Could you check a few things on this model? Use its own coordinates, in mm. A direction names the side the tool comes from. Coordinates: 2 decimals unless noted, no trailing zeros. Order: outer loops, then holes, each group sorted by start corner. A loop starts at its lowest first (then second) coordinate and runs counter-clockwise, first axis right, second up.
```python
from build123d import *

# Parameters (mm, degrees)
SKETCH1_W           = 200
SKETCH1_H           = 110
BOSS_EXTRUDE1_DEPTH = 3.175
CUT_EXTRUDE1_REACH  = 5.175
CUT_EXTRUDE2_REACH  = 5.175
SKETCH4_W           = 6.35
SKETCH4_H           = 25
CUT_EXTRUDE3_DEPTH  = 3.175
SKETCH5_R           = 3.175
CUT_EXTRUDE4_DEPTH  = 10
LPATTERN1_COUNT     = 3
LPATTERN1_PITCH     = 30


with BuildPart() as part:
    # Sketch1 → Boss-Extrude1 (new body)
    with BuildSketch(Plane(origin=(0, 0, 0), x_dir=(1, 0, 0), z_dir=(0, 1, 0))):
        with Locations((100, 55)):
            Rectangle(SKETCH1_W, SKETCH1_H)
    extrude(amount=BOSS_EXTRUDE1_DEPTH)

    # Sketch2 → Cut-Extrude1 (cut, up to next)
    with BuildSketch(Plane(origin=(0, 3.175, 0), x_dir=(1, 0, 0), z_dir=(0, 1, 0)), mode=Mode.PRIVATE) as cut_extrude1_sk1:
        Polygon((194, 22.467727943), (174.625274195, 3.093002139), (170.135146135, 7.583130199), (189.509871939, 26.957856004), align=None)
    cut_extrude1_tool1 = extrude(cut_extrude1_sk1.sketch, amount=-CUT_EXTRUDE1_REACH, mode=Mode.PRIVATE) & part.part
    add(cut_extrude1_tool1.solids().sort_by_distance((182.067573, 3.175, -15.025429))[0], mode=Mode.SUBTRACT)

    # Sketch3 → Cut-Extrude2 (cut, up to next)
    with BuildSketch(Plane(origin=(0, 3.175, 0), x_dir=(1, 0, 0), z_dir=(0, 1, 0)), mode=Mode.PRIVATE) as cut_extrude2_sk1:
        Polygon((168.509871939, 71.151828996), (179.151828996, 60.509871939), (183.641957057, 65), (173, 75.641957057), align=None)
    cut_extrude2_tool1 = extrude(cut_extrude2_sk1.sketch, amount=-CUT_EXTRUDE2_REACH, mode=Mode.PRIVATE) & part.part
    add(cut_extrude2_tool1.solids().sort_by_distance((176.075914, 3.175, -68.075914))[0], mode=Mode.SUBTRACT)

    # Sketch4 → Cut-Extrude3 (cut)
    with BuildSketch(Plane(origin=(0, 3.175, 0), x_dir=(1, 0, 0), z_dir=(0, 1, 0))):
        with Locations((8.175, 24.889181128)):
            Rectangle(SKETCH4_W, SKETCH4_H)
    cut_extrude3 = extrude(amount=-CUT_EXTRUDE3_DEPTH, mode=Mode.SUBTRACT)

    # Sketch5 → Cut-Extrude4 (cut)
    with BuildSketch(Plane(origin=(0, 3.175, 0), x_dir=(1, 0, 0), z_dir=(0, 1, 0))):
        with Locations((8, 102)):
            Circle(SKETCH5_R)
        with Locations((192, 102)):
            Circle(SKETCH5_R)
        with Locations((192, 8)):
            Circle(SKETCH5_R)
        with Locations((8, 8)):
            Circle(SKETCH5_R)
    extrude(amount=-CUT_EXTRUDE4_DEPTH, mode=Mode.SUBTRACT)

    # LPattern1: Cut-Extrude3 ×3
    with Locations(*[(i * LPATTERN1_PITCH, 0, 0) for i in range(1, LPATTERN1_COUNT)]):
        add(cut_extrude3, mode=Mode.SUBTRACT)


solid = part.part
```
Item 1: Which directions (+Z, -Z, +X, -X, +Y, -Y) give clear straight access to the entire face, cutting with the end or side of a thin tool? Please do faces 3 (the face through (99, 0, -56)), 4 (the face through (172.41, 1.61, -5.31)).
Item 2: Suppose I cut it at D-D (z = -35). List the corners of the cut face in (x, y) for me (3 decimals), and give its area (3 significant figures).
Item 3: I need wall thicknesses on line 1 (X direction, y = 2.4, z = -101.5); line 2 (X direction, y = 1.8, z = -102) (3 decimals); line 3 (Z direction, x = 192, y = 1.4) (3 decimals). Which ranges of each line are inside material? Lowest first, please.
Item 4: Suppose I cut it at B-B (x = 8). List the corners of the cut face in (y, z) for me (3 decimals).
Item 5: For pin 1 Ø1 at (x, y) = (7, 1) entering from +Z; pin 2 Ø5 at (x, z) = (192, -8) entering from +Y, each with a flat end and sliding along its axis, tell me the tip position at first contact or that it passes through.
Item 6: Thinking about a two-plate mould opening in Z: for faces 1 (the face through (99, 3.175, -56)), 2 (the face through (184.45, 1.61, -12.92)), which applies, +Z half, -Z half, draft (parallel to the pull), parting line (faces both ways), or undercut?
Item 7: Suppose I cut it at A-A (z = -102). List the corners of the cut face in (x, y) for me (3 decimals).
Item 8: Suppose I cut it at C-C (y = 1.35). Count the separate pieces of the cut face and the enclosed holes in it, and give its area (3 significant figures).
Geometry results:
1. face 3: +Z, -Z, +X, -X, -Y
1. face 4: +Y, -Y
2. outline: (0, 0) - (5, 0) - (5, 3.175) - (0, 3.175) - close; (11.35, 0) - (35, 0) - (35, 3.175) - (11.35, 3.175) - close; (41.35, 0) - (65, 0) - (65, 3.175) - (41.35, 3.175) - close; (71.35, 0) - (200, 0) - (200, 3.175) - (71.35, 3.175) - close
2. area: 575 mm2
3. line 1: x = 0 to 4.86, 11.14 to 188.86, 195.14 to 200
3. line 2: x = 0 to 4.825, 11.175 to 188.825, 195.175 to 200
3. line 3: z = -110 to -105.175, -98.825 to -24.468, -20.468 to -11.175, -4.825 to 0
4. outline: (0, -110) - (3.175, -110) - (3.175, -105.175) - (0, -105.175) - close; (0, -98.825) - (3.175, -98.825) - (3.175, -37.389) - (0, -37.389) - close; (0, -12.389) - (3.175, -12.389) - (3.175, -11.175) - (0, -11.175) - close; (0, -4.825) - (3.175, -4.825) - (3.175, 0) - (0, 0) - close
5. pin 1: stops at z = 0
5. pin 2: passes through
6. face 1: draft
6. face 2: undercut
7. outline: (0, 0) - (4.825, 0) - (4.825, 3.175) - (0, 3.175) - close; (11.175, 0) - (188.825, 0) - (188.825, 3.175) - (11.175, 3.175) - close; (195.175, 0) - (200, 0) - (200, 3.175) - (195.175, 3.175) - close
8. separate pieces: 1
8. enclosed holes: 9
8. area: 21,100 mm2
